Build history of the part. All positions in model axes, mm. A direction names the side the tool comes from. Round coordinates to 2 decimals unless told otherwise and drop trailing zeros. Order: outer loops, then holes, each group sorted by start corner. A loop starts at its lowest first (then second) coordinate and runs counter-clockwise, first axis right, second up. Notation, with made-up numbers: M 12,77 L 22,77 A12 cw 22,81 Z; hole C 5,22 d8. An arc over 180 degrees is marked long. Use CSV: the item, a comma, the result in double quotes.
from build123d import *

# Parameters (mm, degrees)
F0_W     = 196.85
F0_H     = 47.9044
F1_DEPTH = 76.2
F2_R     = 4.7752
F2_R_2   = 1.9812
F3_DEPTH = 47.9054
F5_DEPTH = 31.7246
F7_DEPTH = 16.002
F9_DEPTH = 33.528


with BuildPart() as f1:
    # F0 (on Top) → F1 (new body)
    with BuildSketch(Plane.XY):
        with Locations((-0.5334, 0)):
            Rectangle(F0_W, F0_H)
    extrude(amount=-F1_DEPTH)

    # F2 (on face) → F3 (cut, through all)
    with BuildSketch(Plane.XZ.offset(23.9522)):
        with Locations((-49.9872, -18.1356)):
            Circle(F2_R)
        with Locations((-21.4122, -23.8506)):
            Circle(F2_R_2)
        with Locations((0, -15.875)):
            Circle(F2_R_2)
    extrude(amount=-F3_DEPTH, mode=Mode.SUBTRACT)

    # F4 (on face) → F5 (cut)
    with BuildSketch(Plane.XY):
        with BuildLine():
            ThreePointArc((8.6106, 3.2258), (6.988792, 7.141192), (3.0734, 8.763))
            Line((3.0734, 8.763), (-38.4048, 8.763))
            ThreePointArc((-38.4048, 8.763), (-40.989492, 8.122733), (-42.976447, 6.35))
            Line((-42.976447, 6.35), (-50.8762, 6.35))
            ThreePointArc((-50.8762, 6.35), (-52.702781, 6.040054), (-54.324875, 5.144915))
            ThreePointArc((-54.324875, 5.144915), (-55.864015, 3.217439), (-56.4134, 0.8128))
            Line((-56.4134, 0.8128), (-56.4134, 0.762))
            ThreePointArc((-56.4134, 0.762), (-54.791592, -3.153392), (-50.8762, -4.7752))
            Line((-50.8762, -4.7752), (-43.720808, -4.7752))
            ThreePointArc((-43.720808, -4.7752), (-41.727543, -7.655242), (-38.4048, -8.763))
            Line((-38.4048, -8.763), (3.0734, -8.763))
            ThreePointArc((3.0734, -8.763), (6.988792, -7.141192), (8.6106, -3.2258))
            Line((8.6106, -3.2258), (8.6106, 3.2258))
        make_face()
    extrude(amount=-F5_DEPTH, mode=Mode.SUBTRACT)

    # F6 (on face) → F7 (cut)
    with BuildSketch(Plane.XY):
        with BuildLine():
            Line((-49.2252, 6.35), (-75.057, 6.35))
            ThreePointArc((-75.057, 6.35), (-78.972392, 4.728192), (-80.5942, 0.8128))
            Line((-80.5942, 0.8128), (-80.5942, -0.8128))
            ThreePointArc((-80.5942, -0.8128), (-78.972392, -4.728192), (-75.057, -6.35))
            Line((-75.057, -6.35), (-54.7624, -6.35))
            ThreePointArc((-54.7624, -6.35), (-50.847008, -4.728192), (-49.2252, -0.8128))
            Line((-49.2252, -0.8128), (-49.2252, 6.35))
        make_face()
    extrude(amount=-F7_DEPTH, mode=Mode.SUBTRACT)

    # F8 (on face) → F9 (cut)
    with BuildSketch(Plane.XY):
        with BuildLine():
            Line((-12.1666, 3.9624), (-21.5138, 3.9624))
            ThreePointArc((-21.5138, 3.9624), (-24.31564, 2.80184), (-25.4762, 0))
            ThreePointArc((-25.4762, 0), (-24.31564, -2.80184), (-21.5138, -3.9624))
            Line((-21.5138, -3.9624), (-12.1666, -3.9624))
            ThreePointArc((-12.1666, -3.9624), (-9.36476, -2.80184), (-8.2042, 0))
            ThreePointArc((-8.2042, 0), (-9.36476, 2.80184), (-12.1666, 3.9624))
        make_face()
    extrude(amount=-F9_DEPTH, mode=Mode.SUBTRACT)


solid = f1.part
(1) Two-plate mould, pull along Y, no slides. Class faces 1 (the face through (-40.96, 8.14, -15.64)), 2 (the face through (-18, -8.763, -16)), 3 (the face through (-2, -23.952, -38)), 4 (the face through (97.892, 0, -38)): released by +Y, released by -Y, zero draft, split by the parting line, or undercut.
Answer block:
face 1,"undercut"
face 2,"undercut"
face 3,"released by -Y"
face 4,"zero draft"
(2) Cut at A-A, the plane x = 0. Give the cut face in (y, z), and give its area (3 significant figures).
Answer block:
outline,"M -23.95,-76.2 L 23.95,-76.2 L 23.95,-17.86 L 8.76,-17.86 L 8.76,-31.72 L -8.76,-31.72 L -8.76,-17.86 L -23.95,-17.86 Z; M -23.95,-13.89 L -8.76,-13.89 L -8.76,0 L -23.95,0 Z; M 8.76,-13.89 L 23.95,-13.89 L 23.95,0 L 8.76,0 Z"
area,"2,970 mm²"
(3) Drop flat-ended pins along their axis: pin 1 (6.5 mm diameter, centred on x = -66.5, y = -1.5, fed in from +Z); pin 2 (7.5 mm diameter, centred on x = -49.99, z = -18.14, fed in from +Y); pin 3 (8.5 mm diameter, centred on x = -16.5, y = 0.5, fed in from +Z). Give the stop position or say it passes through.
Answer block:
pin 1,"stops at z = -16"
pin 2,"passes through"
pin 3,"stops at z = -31.72"
(4) Tool access for faces 5 (the face through (-55.45, -2.36, -25.5)), 6 (the face through (-2, -10, 0)): list every direction of +Z, -Z, +X, -X, +Y, -Y with a clear straight run to the whole face (end or side of a thin tool).
Answer block:
face 5,"+Z"
face 6,"+Z, +X, -X, +Y, -Y"
(5) Wall check: line 1 (X direction, y = 18.5, z = -17); line 2 (Z direction, x = 0, y = -14); line 3 (Y direction, x = -0.5, z = -27). Give the ranges that are in metal, low to high. Write a range as from..to.
Answer block:
line 1,"x = -98.96..-54.63, -45.35..-1.63, 1.63..97.89"
line 2,"z = -76.2..-17.86, -13.89..0"
line 3,"y = -23.95..-8.76, 8.76..23.95"
